Geometry check sheet. Reference: the model listing, model coordinates, mm. A direction names the side the tool comes from. Round coordinates to 2 decimals unless told otherwise and drop trailing zeros. Return JSON: item names as keys, results as strings.
```python
from build123d import *

# Parameters (mm, degrees)
SKETCH_10_R                   = 10
SM_BASE_FLANGE_3_DEPTH        = 2
SM_EDGE_FLANGE_6_DEPTH        = 230
SM_EDGE_FLANGE_6_BEND_DEPTH   = 230
SM_EDGE_FLANGE_6_BEND_2_DEPTH = 230
CUT_EXTRUDE_4_REACH           = 363.137
SKETCH_47_R                   = 2
CUT_EXTRUDE_6_REACH           = 263.424
SKETCH_50_R                   = 2
CUT_EXTRUDE_7_REACH           = 351.772
SKETCH_51_R                   = 2
CUT_EXTRUDE_8_REACH           = 349.61
SKETCH_52_R                   = 14
SKETCH_53_R                   = 1.5
CUT_EXTRUDE_9_DEPTH           = 10
OTHER_START                   = -20
OTHER_2_OUTLINE_R             = 1.5
OTHER_2_DEPTH                 = 20


# Read off the part's stored shape, not the designer's step: Полость2
# Sheet-metal steps are written as plain solids
with BuildPart() as part:
    # Эскиз10 → Базовая кромка3 (new body)
    with BuildSketch(Plane.XY):
        Polygon((0, 0), (-21, 36.373066959), (94, 235.558909829), (136, 235.558909829), (251, 36.373066959), (230, 0), align=None)
        with Locations((171.849364905, 123.465988394)):
            Circle(SKETCH_10_R, mode=Mode.SUBTRACT)
    extrude(amount=-SM_BASE_FLANGE_3_DEPTH)

    # Ребро-кромка6 section (across the edge) → Ребро-кромка6 (add)
    with BuildSketch(Plane(origin=(-21.866025404, 36.873066959, -2), x_dir=(0.8660254037844436, -0.4999999999999914, -3.4914813388431334e-15), z_dir=(0.4999999999999914, 0.8660254037844436, 0))):
        with BuildLine():
            Line((-2, 1), (-2, 18))
            Line((-2, 18), (0, 18))
            Line((0, 18), (0, 1))
            ThreePointArc((0, 1), (0.292893219, 0.292893219), (1, 0))
            Line((1, 0), (1, -2))
            ThreePointArc((1, -2), (-1.121320344, -1.121320344), (-2, 1))
        make_face()
    extrude(amount=SM_EDGE_FLANGE_6_DEPTH)

    # Ребро-кромка6 section 2 (across the edge) → Ребро-кромка6 bend (add)
    with BuildSketch(Plane(origin=(136.866025404, 236.058909829, -2), x_dir=(-0.8660254037844363, -0.5000000000000041, -3.4914813388431334e-15), z_dir=(0.5000000000000041, -0.8660254037844363, 0))):
        with BuildLine():
            Line((-2, 1), (-2, 18))
            Line((-2, 18), (0, 18))
            Line((0, 18), (0, 1))
            ThreePointArc((0, 1), (0.292893219, 0.292893219), (1, 0))
            Line((1, 0), (1, -2))
            ThreePointArc((1, -2), (-1.121320344, -1.121320344), (-2, 1))
        make_face()
    extrude(amount=SM_EDGE_FLANGE_6_BEND_DEPTH)

    # Ребро-кромка6 section 3 (across the edge) → Ребро-кромка6 bend 2 (add)
    with BuildSketch(Plane(origin=(230, -1, -2), x_dir=(0, 1, 0), z_dir=(-1, 0, 0))):
        with BuildLine():
            Line((-2, 1), (-2, 18))
            Line((-2, 18), (0, 18))
            Line((0, 18), (0, 1))
            ThreePointArc((0, 1), (0.292893219, 0.292893219), (1, 0))
            Line((1, 0), (1, -2))
            ThreePointArc((1, -2), (-1.121320344, -1.121320344), (-2, 1))
        make_face()
    extrude(amount=SM_EDGE_FLANGE_6_BEND_2_DEPTH)

    # Эскиз47 → Вырез-Вытянуть4 (cut, up to next)
    with BuildSketch(Plane(origin=(-34.098076211, 19.686533479, 0), x_dir=(0, 0, 1), z_dir=(-0.866025403784443, 0.4999999999999925, 3.788649256556814e-15)), mode=Mode.PRIVATE) as cut_extrude_4_sk1:
        with Locations(Location((-11.5, 29, 0), (0, 0, 270))):
            Circle(SKETCH_47_R)
    cut_extrude_4_tool1 = extrude(cut_extrude_4_sk1.sketch, amount=-CUT_EXTRUDE_4_REACH, mode=Mode.PRIVATE) & part.part
    # Эскиз47 → Вырез-Вытянуть4 (cut, up to next)
    with BuildSketch(Plane(origin=(-34.098076211, 19.686533479, 0), x_dir=(0, 0, 1), z_dir=(-0.866025403784443, 0.4999999999999925, 3.788649256556814e-15)), mode=Mode.PRIVATE) as cut_extrude_4_sk2:
        with Locations(Location((-11.5, 39, 0), (0, 0, 270))):
            Circle(SKETCH_47_R)
    cut_extrude_4_tool2 = extrude(cut_extrude_4_sk2.sketch, amount=-CUT_EXTRUDE_4_REACH, mode=Mode.PRIVATE) & part.part
    # Эскиз47 → Вырез-Вытянуть4 (cut, up to next)
    with BuildSketch(Plane(origin=(-34.098076211, 19.686533479, 0), x_dir=(0, 0, 1), z_dir=(-0.866025403784443, 0.4999999999999925, 3.788649256556814e-15)), mode=Mode.PRIVATE) as cut_extrude_4_sk3:
        with Locations(Location((-11.5, 233, 0), (0, 0, 270))):
            Circle(SKETCH_47_R)
    cut_extrude_4_tool3 = extrude(cut_extrude_4_sk3.sketch, amount=-CUT_EXTRUDE_4_REACH, mode=Mode.PRIVATE) & part.part
    # Эскиз47 → Вырез-Вытянуть4 (cut, up to next)
    with BuildSketch(Plane(origin=(-34.098076211, 19.686533479, 0), x_dir=(0, 0, 1), z_dir=(-0.866025403784443, 0.4999999999999925, 3.788649256556814e-15)), mode=Mode.PRIVATE) as cut_extrude_4_sk4:
        with Locations(Location((-11.5, 243, 0), (0, 0, 270))):
            Circle(SKETCH_47_R)
    cut_extrude_4_tool4 = extrude(cut_extrude_4_sk4.sketch, amount=-CUT_EXTRUDE_4_REACH, mode=Mode.PRIVATE) & part.part
    add(cut_extrude_4_tool1.solids().sort_by_distance((-19.598076, 44.80127, -11.5))[0], mode=Mode.SUBTRACT)
    add(cut_extrude_4_tool2.solids().sort_by_distance((-14.598076, 53.461524, -11.5))[0], mode=Mode.SUBTRACT)
    add(cut_extrude_4_tool3.solids().sort_by_distance((82.401924, 221.470453, -11.5))[0], mode=Mode.SUBTRACT)
    add(cut_extrude_4_tool4.solids().sort_by_distance((87.401924, 230.130707, -11.5))[0], mode=Mode.SUBTRACT)

    # Эскиз50 → Вырез-Вытянуть6 (cut, up to next)
    with BuildSketch(Plane(origin=(206.598076211, 119.279454915, 0), x_dir=(0, 0, -1), z_dir=(0.866025403784436, 0.5000000000000047, 3.0623287353932815e-15)), mode=Mode.PRIVATE) as cut_extrude_6_sk1:
        with Locations(Location((11.5, -86, 0), (0, 0, 90))):
            Circle(SKETCH_50_R)
    cut_extrude_6_tool1 = extrude(cut_extrude_6_sk1.sketch, amount=-CUT_EXTRUDE_6_REACH, mode=Mode.PRIVATE) & part.part
    # Эскиз50 → Вырез-Вытянуть6 (cut, up to next)
    with BuildSketch(Plane(origin=(206.598076211, 119.279454915, 0), x_dir=(0, 0, -1), z_dir=(0.866025403784436, 0.5000000000000047, 3.0623287353932815e-15)), mode=Mode.PRIVATE) as cut_extrude_6_sk2:
        with Locations(Location((11.5, -76, 0), (0, 0, 90))):
            Circle(SKETCH_50_R)
    cut_extrude_6_tool2 = extrude(cut_extrude_6_sk2.sketch, amount=-CUT_EXTRUDE_6_REACH, mode=Mode.PRIVATE) & part.part
    # Эскиз50 → Вырез-Вытянуть6 (cut, up to next)
    with BuildSketch(Plane(origin=(206.598076211, 119.279454915, 0), x_dir=(0, 0, -1), z_dir=(0.866025403784436, 0.5000000000000047, 3.0623287353932815e-15)), mode=Mode.PRIVATE) as cut_extrude_6_sk3:
        with Locations(Location((11.5, 118, 0), (0, 0, 90))):
            Circle(SKETCH_50_R)
    cut_extrude_6_tool3 = extrude(cut_extrude_6_sk3.sketch, amount=-CUT_EXTRUDE_6_REACH, mode=Mode.PRIVATE) & part.part
    # Эскиз50 → Вырез-Вытянуть6 (cut, up to next)
    with BuildSketch(Plane(origin=(206.598076211, 119.279454915, 0), x_dir=(0, 0, -1), z_dir=(0.866025403784436, 0.5000000000000047, 3.0623287353932815e-15)), mode=Mode.PRIVATE) as cut_extrude_6_sk4:
        with Locations(Location((11.5, 128, 0), (0, 0, 90))):
            Circle(SKETCH_50_R)
    cut_extrude_6_tool4 = extrude(cut_extrude_6_sk4.sketch, amount=-CUT_EXTRUDE_6_REACH, mode=Mode.PRIVATE) & part.part
    add(cut_extrude_6_tool1.solids().sort_by_distance((249.598076, 44.80127, -11.5))[0], mode=Mode.SUBTRACT)
    add(cut_extrude_6_tool2.solids().sort_by_distance((244.598076, 53.461524, -11.5))[0], mode=Mode.SUBTRACT)
    add(cut_extrude_6_tool3.solids().sort_by_distance((147.598076, 221.470453, -11.5))[0], mode=Mode.SUBTRACT)
    add(cut_extrude_6_tool4.solids().sort_by_distance((142.598076, 230.130707, -11.5))[0], mode=Mode.SUBTRACT)

    # Эскиз51 → Вырез-Вытянуть7 (cut, up to next)
    with BuildSketch(Plane.XZ.offset(3), mode=Mode.PRIVATE) as cut_extrude_7_sk1:
        with Locations(Location((222, -11.5, 0), (0, 0, 270))):
            Circle(SKETCH_51_R)
    cut_extrude_7_tool1 = extrude(cut_extrude_7_sk1.sketch, amount=-CUT_EXTRUDE_7_REACH, mode=Mode.PRIVATE) & part.part
    # Эскиз51 → Вырез-Вытянуть7 (cut, up to next)
    with BuildSketch(Plane.XZ.offset(3), mode=Mode.PRIVATE) as cut_extrude_7_sk2:
        with Locations(Location((212, -11.5, 0), (0, 0, 270))):
            Circle(SKETCH_51_R)
    cut_extrude_7_tool2 = extrude(cut_extrude_7_sk2.sketch, amount=-CUT_EXTRUDE_7_REACH, mode=Mode.PRIVATE) & part.part
    # Эскиз51 → Вырез-Вытянуть7 (cut, up to next)
    with BuildSketch(Plane.XZ.offset(3), mode=Mode.PRIVATE) as cut_extrude_7_sk3:
        with Locations(Location((18, -11.5, 0), (0, 0, 270))):
            Circle(SKETCH_51_R)
    cut_extrude_7_tool3 = extrude(cut_extrude_7_sk3.sketch, amount=-CUT_EXTRUDE_7_REACH, mode=Mode.PRIVATE) & part.part
    # Эскиз51 → Вырез-Вытянуть7 (cut, up to next)
    with BuildSketch(Plane.XZ.offset(3), mode=Mode.PRIVATE) as cut_extrude_7_sk4:
        with Locations(Location((8, -11.5, 0), (0, 0, 270))):
            Circle(SKETCH_51_R)
    cut_extrude_7_tool4 = extrude(cut_extrude_7_sk4.sketch, amount=-CUT_EXTRUDE_7_REACH, mode=Mode.PRIVATE) & part.part
    add(cut_extrude_7_tool1.solids().sort_by_distance((222, -3, -11.5))[0], mode=Mode.SUBTRACT)
    add(cut_extrude_7_tool2.solids().sort_by_distance((212, -3, -11.5))[0], mode=Mode.SUBTRACT)
    add(cut_extrude_7_tool3.solids().sort_by_distance((18, -3, -11.5))[0], mode=Mode.SUBTRACT)
    add(cut_extrude_7_tool4.solids().sort_by_distance((8, -3, -11.5))[0], mode=Mode.SUBTRACT)

    # Эскиз52 → Вырез-Вытянуть8 (cut, up to next)
    with BuildSketch(Plane(origin=(0, 0, -2), x_dir=(-1, 0, 0), z_dir=(0, 0, -1)), mode=Mode.PRIVATE) as cut_extrude_8_sk1:
        with Locations((-115, 90.643992263)):
            Circle(SKETCH_52_R)
    cut_extrude_8_tool1 = extrude(cut_extrude_8_sk1.sketch, amount=-CUT_EXTRUDE_8_REACH, mode=Mode.PRIVATE) & part.part
    add(cut_extrude_8_tool1.solids().sort_by_distance((115, 90.643992, -2))[0], mode=Mode.SUBTRACT)

    # Эскиз53 → Вырез-Вытянуть9 (cut)
    with BuildSketch(Plane(origin=(0, 0, -2), x_dir=(-1, 0, 0), z_dir=(0, 0, -1))):
        with Locations((-40.121778265, 70.507041555)):
            Circle(SKETCH_53_R)
        with Locations((-22.801270189, 60.507041555)):
            Circle(SKETCH_53_R)
        with Locations((-60.121778265, 35.866025404)):
            Circle(SKETCH_53_R)
        with Locations((-42.801270189, 25.866025404)):
            Circle(SKETCH_53_R)
        with Locations((-95, 185.558909829)):
            Circle(SKETCH_53_R)
        with Locations((-95, 165.558909829)):
            Circle(SKETCH_53_R)
        with Locations((-135, 185.558909829)):
            Circle(SKETCH_53_R)
        with Locations((-135, 165.558909829)):
            Circle(SKETCH_53_R)
        with Locations((-207.198729811, 60.507041555)):
            Circle(SKETCH_53_R)
        with Locations((-189.878221735, 70.507041555)):
            Circle(SKETCH_53_R)
        with Locations((-187.198729811, 25.866025404)):
            Circle(SKETCH_53_R)
        with Locations((-169.878221735, 35.866025404)):
            Circle(SKETCH_53_R)
    extrude(amount=-CUT_EXTRUDE_9_DEPTH, mode=Mode.SUBTRACT)

    # Полость2 outline → Полость2 (cut)
    with BuildSketch(Plane.XY.offset(OTHER_START)):
        with BuildLine():
            Line((115.008517475, 104.643989672), (115.008517475, 235.558909829))
            Line((115.008517475, 235.558909829), (94, 235.558909829))
            Line((94, 235.558909829), (91.401923789, 237.058909829))
            Line((91.401923789, 237.058909829), (-23.598076211, 37.873066959))
            Line((-23.598076211, 37.873066959), (-21, 36.373066959))
            Line((-21, 36.373066959), (0, 0))
            Line((0, 0), (0, -3))
            Line((0, -3), (230, -3))
            Line((230, -3), (230, 0))
            Line((230, 0), (240.504258738, 18.193909829))
            Line((240.504258738, 18.193909829), (127.128612147, 83.651369908))
            ThreePointArc((127.128612147, 83.651369908), (102.875644347, 83.643992263), (115.008517475, 104.643989672))
        make_face()
        with Locations((42.801270189, 25.866025404)):
            Circle(OTHER_2_OUTLINE_R, mode=Mode.SUBTRACT)
        with Locations((60.121778265, 35.866025404)):
            Circle(OTHER_2_OUTLINE_R, mode=Mode.SUBTRACT)
        with Locations((22.801270189, 60.507041555)):
            Circle(OTHER_2_OUTLINE_R, mode=Mode.SUBTRACT)
        with Locations((40.121778265, 70.507041555)):
            Circle(OTHER_2_OUTLINE_R, mode=Mode.SUBTRACT)
        with Locations((169.878221735, 35.866025404)):
            Circle(OTHER_2_OUTLINE_R, mode=Mode.SUBTRACT)
        with Locations((187.198729811, 25.866025404)):
            Circle(OTHER_2_OUTLINE_R, mode=Mode.SUBTRACT)
        with Locations((95, 165.558909829)):
            Circle(OTHER_2_OUTLINE_R, mode=Mode.SUBTRACT)
        with Locations((95, 185.558909829)):
            Circle(OTHER_2_OUTLINE_R, mode=Mode.SUBTRACT)
    extrude(amount=OTHER_2_DEPTH, mode=Mode.SUBTRACT)


solid = part.part
```
(1) Gauge pin test, flat ends, axial feed: pin 1 (6 mm diameter, centred on x = 148.5, z = -3, fed in from -Y); pin 2 (4 mm diameter, centred on x = 131, y = 99.5, fed in from -Z); pin 3 (4 mm diameter, centred on x = 135, y = 165.56, fed in from +Z); pin 4 (12 mm diameter, centred on x = 210.5, z = -17, fed in from +Y). Record the tip position at first contact, or that the pin passes through.
Response values:
{"pin 1": "stops at y = 69.68", "pin 2": "stops at z = -2", "pin 3": "stops at z = 0", "pin 4": "stops at y = 122.91"}
(2) Material ranges on line 1 along Y through (x, z) = (135, -1.25); line 2 along Z through (x, y) = (185.5, 110.5); line 3 along X through (y, z) = (107, -10.5), recorded low to high. Write a range as [from, to].
Response values:
{"line 1": "y = [79.11, 164.06], [167.06, 184.06], [187.06, 235.56]", "line 2": "z = [-2, 0]", "line 3": "x = [211.38, 213.69]"}
(3) Access from +Z, -Z, +X, -X, +Y, -Y to the whole of each face (thin tool, end or side, straight path). Record for faces 4 (the face through (127.02, 97.82, -1.01)), 5 (the face through (193.56, 137.86, -11.62)).
Response values:
{"face 4": "+Z, -Z, -X", "face 5": "-Z, -X, -Y"}
(4) Release check for a two-part mould opening along Z. For faces 1 (the face through (184.61, 50.464, -1.014)), 2 (the face through (142.48, 228.36, -10.15)), 3 (the face through (194, 138, -20)) record: pulls with the +Z half, pulls with the -Z half, needs draft (parallel to the pull), parting line crosses it, or undercut.
Response values:
{"face 1": "needs draft", "face 2": "undercut", "face 3": "pulls with the -Z half"}
